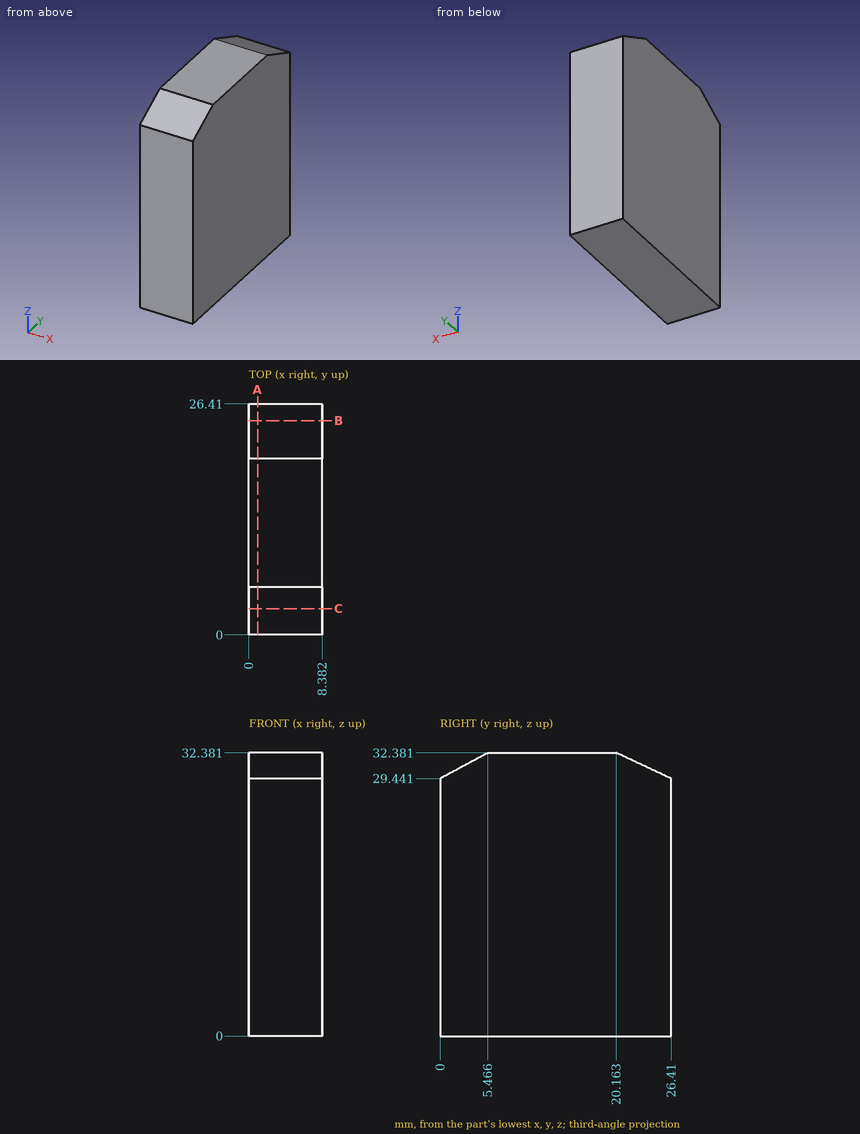
Could you check a few things on this drawing? It's one solid part, dimensions in mm from its lowest x, y, z. Give positions to 0.01 mm unless a question says otherwise; leave off trailing zeros. Write each loop counter-clockwise with the first axis right and the second up, starting at its lowest first coordinate (ties: lowest second). Pieces come first, ordered by that corner, then holes. Notation, with made-up numbers: (18, 67) -> (45, 67) arc R21 ccw to (45, 106) -> close; hole circle Ø7 at (-39.5, 1.25). An arc over 180 degrees is marked (long way). Write item = value, one per line.
(1) Suppose I cut it at C-C on y = 3. Write out the boundary of the cut face in (x, z) (1 decimal), then the cut area to 3 significant figures.
Worked out:
outline = (0, 0) -> (8.4, 0) -> (8.4, 31.1) -> (0, 31.1) -> close
area = 260 mm^2
(2) Suppose I cut it at B-B on y = 24.5. Write out the boundary of the cut face in (x, z).
Worked out:
outline = (0, 0) -> (8.38, 0) -> (8.38, 30.34) -> (0, 30.34) -> close
(3) Suppose I cut it at A-A on x = 1. Write out the boundary of the cut face in (y, z) (1 decimal).
Worked out:
outline = (0, 0) -> (26.4, 0) -> (26.4, 29.4) -> (20.2, 32.4) -> (5.5, 32.4) -> (0, 29.4) -> close
(4) I need wall thicknesses on probe 1 along Z at (x, y) = (6, 21); probe 2 along Z at (x, y) = (6.5, 2.25). Which ranges of each line are inside material? Lowest first, please. Write a range as from..to.
Worked out:
probe_1 = 0..31.99
probe_2 = 0..30.65
